The listing builds one solid part. Answer for the finished solid, in the listing's coordinates (mm). Face numbers are marked on the shaded views. A direction names the side the tool comes from. Round coordinates to 2 decimals unless told otherwise and drop trailing zeros. Order: outer loops, then holes, each group sorted by start corner. A loop starts at its lowest first (then second) coordinate and runs counter-clockwise, first axis right, second up. Notation, with made-up numbers: (70, 37.5) - (118, 37.5) arc R25 ccw to (118, 50.5) - close; hole circle Ø2 at (-24, -24.5). An arc over 180 degrees is marked (long way). One line per item, written item: value. Start each with the question number.
1. Section C-C, the plane x = -40 is taken. Give the vertices of the cut face in (y, z).
2. For a pull along Z with two mould halves and no side action, classify the marked faces 5, 6 and 7 as released by +Z, released by -Z, zero draft, split by the parting line, or undercut.
3. Flat-ended cylindrical pins translate along their axes: P1, Ø7, axis at y = 1.5, z = -8.5, coming from the +X side (3 decimals); P2, Ø1.8, axis at x = 27, y = 4, coming from the +Z side; P3, Ø1.5, axis at y = -1, z = -16, coming from the -X side. Find the tip coordinate at first contact, or state that the pin passes through.
4. Section A-A, the plane x = 0 is taken. Give the vertices of the cut face in (y, z).
5. Section D-D, the plane x = 34 is taken. Give the vertices of the cut face in (y, z), then the cut area to 3 significant figures.
6. Straight lines are drawn through the part: line 1 (X direction, y = 1.65, z = 0); line 2 (Y direction, x = 42, z = -6.5); line 3 (X direction, y = 4, z = 5) (1 decimal). For each, find the intervals that lie inside material, in ascending order.
7. A tool of negligible diameter and unlimited length cuts with its end or side. For the marked faces 1, 2, 3 and 4, from which of +Z, -Z, +X, -X, +Y, -Y can it reach the whole face along a straight path? Write none if from no direction.
8. Section B-B, the plane z = 0 is taken. Give the vertices of the cut face in (x, y).
from build123d import *

# Parameters (mm, degrees)
ESBO_O1_R                     = 4.05
ESBO_O1_R_2                   = 11.4
RESSALTO_EXTRUS_O1_DEPTH      = 6
RESSALTO_EXTRUS_O2_START      = -1
ESBO_O2_R                     = 11.4
ESBO_O2_R_2                   = 10.65
RESSALTO_EXTRUS_O2_DEPTH      = 1
RESSALTO_EXTRUS_O4_DEPTH      = 3
RESSALTO_EXTRUS_O4_DEPTH_BACK = 5.673111
ESBO_O4_R                     = 4.15
CHANFRO1_SIZE                 = 2.360185131
CHANFRO1_SIZE_2               = 3


with BuildPart() as part:
    # Esboço1 → Ressalto-extrusão1 (new body)
    with BuildSketch(Plane(origin=(0, 0, 0), x_dir=(1, 0, 0), z_dir=(0, 1, 0))):
        with BuildLine():
            Line((-33.07179677, 4), (-28, 4))
            Line((-28, 4), (-28, 19))
            Line((-28, 19), (-22, 19))
            Line((-22, 19), (-22, 4))
            Line((-22, 4), (-21.193395198, 4))
            ThreePointArc((-21.193395198, 4), (-16.456207753, 5.193238103), (-12.849538821, 8.488188976))
            ThreePointArc((-12.849538821, 8.488188976), (0, 15.4), (12.849538821, 8.488188976))
            ThreePointArc((12.849538821, 8.488188976), (16.456207753, 5.193238103), (21.193395198, 4))
            Line((21.193395198, 4), (33.07179677, 4))
            ThreePointArc((33.07179677, 4), (48, 0), (33.07179677, -4))
            Line((33.07179677, -4), (21.193395198, -4))
            ThreePointArc((21.193395198, -4), (16.456207753, -5.193238103), (12.849538821, -8.488188976))
            ThreePointArc((12.849538821, -8.488188976), (0, -15.4), (-12.849538821, -8.488188976))
            ThreePointArc((-12.849538821, -8.488188976), (-16.456207753, -5.193238103), (-21.193395198, -4))
            Line((-21.193395198, -4), (-33.07179677, -4))
            ThreePointArc((-33.07179677, -4), (-48, 0), (-33.07179677, 4))
        make_face()
        with Locations(Location((40, 0, 0), (0, 0, 270))):
            Circle(ESBO_O1_R, mode=Mode.SUBTRACT)
        with Locations(Location((-40, 0, 0), (0, 0, 270))):
            Circle(ESBO_O1_R, mode=Mode.SUBTRACT)
        with Locations(Location((0, 0, 0), (0, 0, 270))):
            Circle(ESBO_O1_R_2, mode=Mode.SUBTRACT)
    extrude(amount=RESSALTO_EXTRUS_O1_DEPTH)

    # Esboço2 → Ressalto-extrusão2 (add)
    with BuildSketch(Plane(origin=(0, 6, 0), x_dir=(1, 0, 0), z_dir=(0, 1, 0)).offset(RESSALTO_EXTRUS_O2_START)):
        with Locations(Location((0, 0, 0), (0, 0, 270))):
            Circle(ESBO_O2_R)
        with Locations(Location((0, 0, 0), (0, 0, 270))):
            Circle(ESBO_O2_R_2, mode=Mode.SUBTRACT)
    extrude(amount=RESSALTO_EXTRUS_O2_DEPTH)

    # Esboço4 → Ressalto-extrusão4 (add, two sides: drawn at the far end of the back side and taken through both)
    with BuildSketch(Plane(origin=(0, 5.848784016, -2.013897841), x_dir=(-1, 0, 0), z_dir=(0, -0.9455185755993178, 0.32556815445715404)).offset(-RESSALTO_EXTRUS_O4_DEPTH_BACK)):
        with BuildLine():
            Line((28, 16.01144401), (22, 16.01144401))
            Line((22, 16.01144401), (22, 17.964852936))
            ThreePointArc((22, 17.964852936), (25, 31.289408257), (28, 17.964852936))
            Line((28, 17.964852936), (28, 16.01144401))
        make_face()
        with Locations(Location((25, 24.289408257, 0), (0, 0, 90))):
            Circle(ESBO_O4_R, mode=Mode.SUBTRACT)
    extrude(amount=RESSALTO_EXTRUS_O4_DEPTH + RESSALTO_EXTRUS_O4_DEPTH_BACK)

    # Chanfro1
    # the kernel refuses this chamfer: 3, 2.360185131 mm, written as the material it adds along each edge
    with BuildSketch(Plane(origin=(-22, 0, -16.93403432), x_dir=(0, -0.9591141724296175, 0.28301944146056485), z_dir=(-1, 0, 0))) as chanfro1_piece_1_section:
        Polygon((CHANFRO1_SIZE * 0.999002383221, CHANFRO1_SIZE * 0.0446568918676), (CHANFRO1_SIZE_2 * 0.283019441461, CHANFRO1_SIZE_2 * 0.95911417243), (0, 0), align=None)
    chanfro1_piece_1 = extrude(amount=6, mode=Mode.PRIVATE)
    chanfro1_piece_1 = split(chanfro1_piece_1, bisect_by=Plane(origin=(-25, -1.892415704, -15.281313813), z_dir=(0, 0.9455185755993178, -0.32556815445715404)), keep=Keep.TOP, mode=Mode.PRIVATE)
    add(chanfro1_piece_1)


solid = part.part
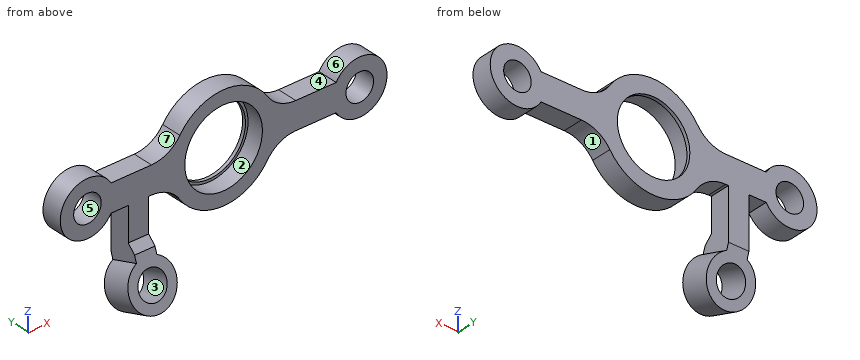
Answer list:
1. outline: (0, -8) - (6, -8) - (6, -4.05) - (0, -4.05) - close; (0, 4.05) - (6, 4.05) - (6, 8) - (0, 8) - close
2. face 5: undercut
2. face 6: split by the parting line
2. face 7: released by +Z
3. P1: stops at x = 46.245
3. P2: stops at z = 4
3. P3: stops at x = -28
4. outline: (0, -15.4) - (6, -15.4) - (6, -10.65) - (5, -10.65) - (5, -11.4) - (0, -11.4) - close; (0, 11.4) - (5, 11.4) - (5, 10.65) - (6, 10.65) - (6, 15.4) - (0, 15.4) - close
5. outline: (0, -5.29) - (6, -5.29) - (6, 5.29) - (0, 5.29) - close
5. area: 63.5 mm²
6. line 1: x = -48 to -44.05, -35.95 to -11.4, 11.4 to 35.95, 44.05 to 48
6. line 2: y = 0 to 6
6. line 3: x = -46.2 to -33.8, -16.8 to -10.2, 10.2 to 16.8, 33.8 to 46.2
7. face 1: -Z, +Y, -Y
7. face 2: -Y
7. face 3: none
7. face 4: +Z, +Y, -Y
8. outline: (-48, 0) - (-44.05, 0) - (-44.05, 6) - (-48, 6) - close; (-35.95, 0) - (-11.4, 0) - (-11.4, 5) - (-10.65, 5) - (-10.65, 6) - (-35.95, 6) - close; (10.65, 5) - (11.4, 5) - (11.4, 0) - (35.95, 0) - (35.95, 6) - (10.65, 6) - close; (44.05, 0) - (48, 0) - (48, 6) - (44.05, 6) - close
